from build123d import *
from build123d.topology import SkipClean

# Parameters (mm, degrees)
SKETCH1_R           = 1.75
SKETCH1_R_2         = 5
BOSS_EXTRUDE1_DEPTH = 8
SKETCH2_R           = 22
SKETCH2_R_2         = 1.75
BOSS_EXTRUDE2_DEPTH = 3
SKETCH3_R           = 3.25
SKETCH3_R_2         = 1.75
CUT_EXTRUDE1_DEPTH  = 4


with BuildPart() as part:
    # Sketch1 → Boss-Extrude1 (new body)
    with BuildSketch(Plane(origin=(0, 0, 0), x_dir=(1, 0, 0), z_dir=(0, 1, 0))):
        with BuildLine():
            Line((-150, 12.5), (0, 22))
            ThreePointArc((0, 22), (22, 0), (0, -22))
            Line((0, -22), (-150, -12.5))
            ThreePointArc((-150, -12.5), (-162.5, 0), (-150, 12.5))
        make_face()
        with Locations(Location((0, 17, 0), (0, 0, 270))):
            Circle(SKETCH1_R, mode=Mode.SUBTRACT)
        with Locations(Location((17, 0, 0), (0, 0, 270))):
            Circle(SKETCH1_R, mode=Mode.SUBTRACT)
        with Locations(Location((0, -17, 0), (0, 0, 270))):
            Circle(SKETCH1_R, mode=Mode.SUBTRACT)
        with Locations(Location((-17, 0, 0), (0, 0, 270))):
            Circle(SKETCH1_R, mode=Mode.SUBTRACT)
        with Locations(Location((-150, 0, 0), (0, 0, 270))):
            Circle(SKETCH1_R_2, mode=Mode.SUBTRACT)
    extrude(amount=BOSS_EXTRUDE1_DEPTH)

    # Sketch2 → Boss-Extrude2 (add)
    with SkipClean():  # the faces are left unmerged after this step: merging them gives an invalid solid
        with BuildSketch(Plane(origin=(0, 8, 0), x_dir=(1, 0, 0), z_dir=(0, 1, 0))):
            with Locations(Location((0, 0, 0), (0, 0, 270))):
                Circle(SKETCH2_R)
            with Locations(Location((-17, 0, 0), (0, 0, 270))):
                Circle(SKETCH2_R_2, mode=Mode.SUBTRACT)
            with Locations(Location((0, -17, 0), (0, 0, 270))):
                Circle(SKETCH2_R_2, mode=Mode.SUBTRACT)
            with Locations(Location((17, 0, 0), (0, 0, 270))):
                Circle(SKETCH2_R_2, mode=Mode.SUBTRACT)
            with Locations(Location((0, 17, 0), (0, 0, 270))):
                Circle(SKETCH2_R_2, mode=Mode.SUBTRACT)
        extrude(amount=BOSS_EXTRUDE2_DEPTH)
    add(part.part.scale(1), mode=Mode.REPLACE)  # the faces are merged on a copy

    # Sketch3 → Cut-Extrude1 (cut)
    # profile 1 of 4: a face of its own
    with BuildSketch(Plane(origin=(0, 0, 0), x_dir=(-1, 0, 0), z_dir=(0, -1, 0))):
        with Locations(Location((0, 17, 0), (0, 0, 90))):
            Circle(SKETCH3_R)
        with Locations(Location((0, 17, 0), (0, 0, 90))):
            Circle(SKETCH3_R_2, mode=Mode.SUBTRACT)
    # profile 2 of 4: a face of its own
    with BuildSketch(Plane(origin=(0, 0, 0), x_dir=(-1, 0, 0), z_dir=(0, -1, 0))):
        with Locations(Location((-17, 0, 0), (0, 0, 90))):
            Circle(SKETCH3_R)
        with Locations(Location((-17, 0, 0), (0, 0, 90))):
            Circle(SKETCH3_R_2, mode=Mode.SUBTRACT)
    # profile 3 of 4: a face of its own
    with BuildSketch(Plane(origin=(0, 0, 0), x_dir=(-1, 0, 0), z_dir=(0, -1, 0))):
        with Locations(Location((0, -17, 0), (0, 0, 90))):
            Circle(SKETCH3_R)
        with Locations(Location((0, -17, 0), (0, 0, 90))):
            Circle(SKETCH3_R_2, mode=Mode.SUBTRACT)
    # profile 4 of 4: a face of its own
    with BuildSketch(Plane(origin=(0, 0, 0), x_dir=(-1, 0, 0), z_dir=(0, -1, 0))):
        with Locations(Location((17, 0, 0), (0, 0, 90))):
            Circle(SKETCH3_R)
        with Locations(Location((17, 0, 0), (0, 0, 90))):
            Circle(SKETCH3_R_2, mode=Mode.SUBTRACT)
    extrude(amount=-CUT_EXTRUDE1_DEPTH, mode=Mode.SUBTRACT)


solid = part.part
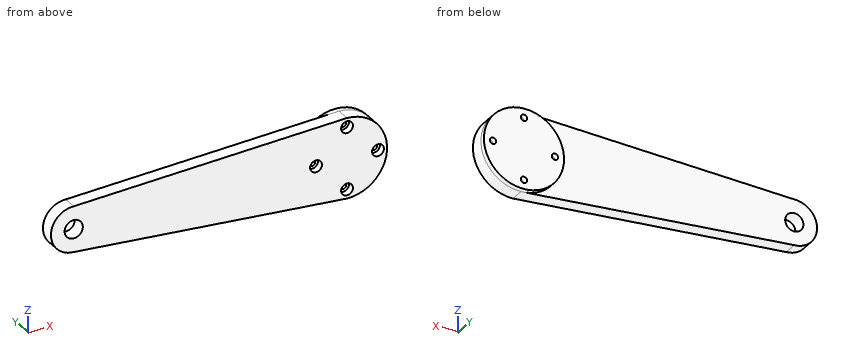
Can you work these out from the model? Positions are in its coordinate system, mm. Give positions to 0.01 mm unless a question says otherwise; leave off trailing zeros. Loops run counter-clockwise (first coordinate to the right, second up) from the corner with the lowest first, then second, coordinate; pieces in that order, holes last. Notation, with made-up numbers: (15.25, 34) - (50.25, 34) arc R22 ccw to (50.25, 52) - close; hole circle Ø9 at (68, -15.75). An arc over 180 degrees is marked (long way). Answer as a JSON object with one key per item and string values.
Q1. Imagine slicing it at C-C on x = -17. Write out the boundary of the cut face in (y, z), plus the area to 3 significant figures.
Geometry says:
{"outline": "(0, -20.92) - (8, -20.92) - (8, -13.96) - (11, -13.96) - (11, -1.75) - (4, -1.75) - (4, -3.25) - (0, -3.25) - close; (0, 3.25) - (4, 3.25) - (4, 1.75) - (11, 1.75) - (11, 13.96) - (8, 13.96) - (8, 20.92) - (0, 20.92) - close", "area": "368 mm²"}
Q2. Will these pins go through, and if not, where does the flat tip stop? P1, Ø3, axis at x = -17, z = 0, coming from the -Y side; P2, Ø6, axis at x = 0, z = -17, coming from the +Y side; P3, Ø6, axis at x = 0, z = 17, coming from the -Y side; P4, Ø8, axis at x = -73, z = 4, coming from the +Y side.
Geometry says:
{"P1": "through", "P2": "y = 11", "P3": "y = 4", "P4": "y = 8"}
Q3. Imagine slicing it at B-B on z = -17. Write out the boundary of the cut face in (x, y).
Geometry says:
{"outline": "(-78.95, 0) - (-3.25, 0) - (-3.25, 4) - (-1.75, 4) - (-1.75, 11) - (-13.96, 11) - (-13.96, 8) - (-78.95, 8) - close; (1.75, 4) - (3.25, 4) - (3.25, 0) - (13.96, 0) - (13.96, 11) - (1.75, 11) - close"}
Q4. Imagine slicing it at A-A on x = 17. Write out the boundary of the cut face in (y, z).
Geometry says:
{"outline": "(0, -13.96) - (11, -13.96) - (11, -1.75) - (4, -1.75) - (4, -3.25) - (0, -3.25) - close; (0, 3.25) - (4, 3.25) - (4, 1.75) - (11, 1.75) - (11, 13.96) - (0, 13.96) - close"}
Q5. If I drill on L1, parallel to Z at x = 0, y = 6.8; L2, parallel to X at y = 1.85, z = 0, over which ranges is the centre line in solid material (lowest first)?
Geometry says:
{"L1": "-22 to -18.75, -15.25 to 15.25, 18.75 to 22", "L2": "-162.5 to -155, -145 to -20.25, -13.75 to 13.75, 20.25 to 22"}
Q6. Imagine slicing it at D-D on z = -9. Write out the boundary of the cut face in (x, y).
Geometry says:
{"outline": "(-158.67, 0) - (20.07, 0) - (20.07, 11) - (-20.07, 11) - (-20.07, 8) - (-158.67, 8) - close"}
